The model under review builds one solid part; all positions refer to its coordinate system, in mm. A direction names the side the tool comes from. Round coordinates to 2 decimals unless told otherwise and drop trailing zeros. Write each loop counter-clockwise with the first axis right and the second up, starting at its lowest first coordinate (ties: lowest second). Pieces come first, ordered by that corner, then holes. Notation, with made-up numbers: (78.5, 89) -> (107.5, 89) arc R31 cw to (107.5, 113) -> close; hole circle Ø8 at (68.5, 10). An arc over 180 degrees is marked (long way). Return JSON: item names as keys, results as strings. Group by question number.
1. Take a section at C-C, the plane x = 8.5. Write out the cut boundary in (y, z), then the cut area to 3 significant figures.
2. Take a section at D-D, the plane y = -6.5. Write out the cut boundary in (x, z).
3. Take a section at A-A, the plane y = 16. Write out the cut boundary in (x, z).
4. Take a section at B-B, the plane z = 3.5. Write out the cut boundary in (x, y).
5. Tool access review of faces 1 (the cylindrical face through (-13.092, 23.504, 10.824)), 2 (the cylindrical face through (-13.09, 23.41, 1.7)), 3 (the flat face through (0, 2, 12.7)): name each direction out of +Z, -Z, +X, -X, +Y, -Y from which nothing blocks a thin tool from reaching the whole face with its end or side.
6. For line 1 along X through (y, z) = (20, 1.25); line 2 along Z through (x, y) = (-9, -8.5); line 3 along X through (y, z) = (-20.5, 5.75), list the stretches that pass through material, from the lowest coordinate up. Write a range as from..to.
7. Clearance check with flat-ended pins moving along their axes: P1, Ø0.8, axis at x = -13.5, y = 15.5, coming from the +Z side; P2, Ø4, axis at x = -7, y = 9.5, coming from the -Z side; P3, Ø1.5, axis at y = 9.5, z = 2.5, coming from the +X side. State where each tip first meets the part, or that it passes through.
from build123d import *

# Parameters (mm, degrees)
F1_DEPTH = 12.7
F4_DEPTH = 12.7
F5_W     = 2.54
F5_H     = 12.7
F5_H_2   = 12.6950503836
F6_DEPTH = 12.7
F7_R     = 1.27
F8_DEPTH = 41.148
F9_R     = 6.096
F10_R    = 6.096


with BuildPart() as f1:
    # F0 (on Top) → F1 (new body)
    with BuildSketch(Plane.XY):
        Polygon((16.375921394, 19.4162096841), (-25.0028915287, 4.4738590955), (8.6269701347, -23.8900687796), align=None)
    extrude(amount=F1_DEPTH)


with BuildPart() as f4:
    # F3 (on Top) → F4 (new body)
    with BuildSketch(Plane.XY):
        Polygon((0.3085586267, -25.3981257492), (21.841142794, 12.9662824839), (-22.1497014207, 12.4318432653), align=None)
    extrude(amount=F4_DEPTH)

    # F5 (on face) → F6 (join)
    with BuildSketch(Plane(origin=(-0.1542793134, 12.6990628746, 0), x_dir=(-0.9999262106, -0.0121479774, 0), z_dir=(-0.0121479774, 0.9999262106, 0))):
        with Locations((-15.151783279, 6.35)):
            Rectangle(F5_W, F5_H)
        with Locations((12.788216721, 6.3096207778)):
            Rectangle(F5_W, F5_H_2)
    extrude(amount=F6_DEPTH)

    # F7 (on face) → F8 (cut)
    with BuildSketch(Plane(origin=(-14.0571793737, -0.1707788994, 0), x_dir=(0.0121479774, -0.9999262106, 0), z_dir=(-0.9999262106, -0.0121479774, 0))):
        with Locations((-19.0405060285, 6.3191110491)):
            Circle(F7_R)
    extrude(amount=-F8_DEPTH, mode=Mode.SUBTRACT)

    # F9
    f9_edges = [f4.edges().sort_by_distance(p)[0] for p in [
        (-13.095832, 25.242775, 12.657146),
        (-13.095832, 25.242775, -0.037904),
    ]]
    fillet(f9_edges, radius=F9_R)

    # F10
    f10_edges = [f4.edges().sort_by_distance(p)[0] for p in [
        (14.842107, 25.582189, 12.7),
        (14.842107, 25.582189, 0),
    ]]
    fillet(f10_edges, radius=F10_R)


solid = f4.part
Output:
{
 "1": {"outline": "(-10.8, 0) -> (12.8, 0) -> (12.8, 12.7) -> (-10.8, 12.7) -> close", "area": "300 mm^2"},
 "2": {"outline": "(-10.91, 0) -> (10.92, 0) -> (10.92, 12.7) -> (-10.91, 12.7) -> close"},
 "3": {"outline": "(-14.25, -0.04) -> (-11.71, -0.04) -> (-11.71, 12.66) -> (-14.25, 12.66) -> close; (13.69, 0) -> (16.23, 0) -> (16.23, 12.7) -> (13.69, 12.7) -> close"},
 "4": {"outline": "(-22.15, 12.43) -> (0.31, -25.4) -> (21.84, 12.97) -> (16.27, 12.9) -> (16.12, 25.02) -> (13.58, 24.99) -> (13.73, 12.87) -> (-11.67, 12.56) -> (-11.82, 24.7) -> (-14.36, 24.66) -> (-14.21, 12.53) -> close"},
 "5": {"face 1": "+Z, -X, +Y", "face 2": "-Z, -X, +Y", "face 3": "+Z, +X, -X, +Y, -Y"},
 "6": {"line 1": "x = -14.3..-11.76, 13.64..16.18", "line 2": "z = 0..12.7", "line 3": "x = -2.6..3.06"},
 "7": {"P1": "stops at z = 12.66", "P2": "stops at z = 0", "P3": "stops at x = 20.32"}
}
